from build123d import *

# Parameters (mm, degrees)
F0_W     = 50
F0_H     = 36
F1_DEPTH = 2
F2_W     = 50
F2_H     = 36
F2_W_2   = 46
F2_H_2   = 32
F3_DEPTH = 4
F4_W     = 2
F4_H     = 36
F5_DEPTH = 85
F6_W     = 50
F6_H     = 36
F7_DEPTH = 3
F8_W     = 46
F8_H     = 32
F9_DEPTH = 25


with BuildPart() as f1:
    # F0 (on Top) → F1 (new body)
    with BuildSketch(Plane.XY):
        with Locations((-32.9025480896, 24.3834912755)):
            Rectangle(F0_W, F0_H)
    extrude(amount=F1_DEPTH)

    # F2 (on face) → F3 (join)
    with BuildSketch(Plane.XY.offset(2)):
        with Locations((-32.9025480896, 24.3834912755)):
            Rectangle(F2_W, F2_H)
        with Locations((-32.9025480896, 24.3834912755)):
            Rectangle(F2_W_2, F2_H_2, mode=Mode.SUBTRACT)
    extrude(amount=F3_DEPTH)

    # F4 (on face) → F5 (join)
    with BuildSketch(Plane.XY.offset(6)):
        with Locations((-56.9025480896, 24.3834912755)):
            Rectangle(F4_W, F4_H)
        with Locations((-8.9025480896, 24.3834912755)):
            Rectangle(F4_W, F4_H)
    extrude(amount=F5_DEPTH)

    # F6 (on face) → F7 (join)
    with BuildSketch(Plane.XY.offset(91)):
        with Locations((-32.9025480896, 24.3834912755)):
            Rectangle(F6_W, F6_H)
    extrude(amount=-F7_DEPTH)

    # F8 (on face) → F9 (cut)
    with BuildSketch(Plane(origin=(0, 0, 88), x_dir=(1, 0, 0), z_dir=(0, 0, -1))):
        with Locations((-32.9025480896, -24.3834912755)):
            Rectangle(F8_W, F8_H)
    extrude(amount=-F9_DEPTH, mode=Mode.SUBTRACT)


solid = f1.part
Work out the finished part from the listing and answer in its coordinate system (mm). A direction names the side the tool comes from. Round coordinates to 2 decimals unless told otherwise and drop trailing zeros. Loops run counter-clockwise (first coordinate to the right, second up) from the corner with the lowest first, then second, coordinate; pieces in that order, holes last. Notation, with made-up numbers: (-20.5, 78.25) - (36.5, 78.25) arc R12 ccw to (36.5, 86.25) - close; hole circle Ø7 at (60, 28). An arc over 180 degrees is marked (long way). Use one line per item in the form item = value. Start each with the question number.
(1) Which of the six approach directions +Z, -Z, +X, -X, +Y, -Y give full straight-line access (tool end or side, diameter ignored) to faces 1 (the face through (-33, 7, 6)), 2 (the face through (-57, 42.383, 39)), 3 (the face through (-33, 40.383, 4))?
(2) Determine the mould class of faces 4 (the face through (-33, 40.383, 89)), 5 (the face through (-33, 25, 0)), 6 (the face through (-33, 41, 88)), 7 (the face through (-33, 41, 6)) for opening direction Z: +Z half, -Z half, draft (parallel to the pull), parting line (faces both ways), or undercut.
(3) Find section A-A on z = 80. Determine the outline of the cut face in (x, y), and give its area (3 significant figures).
(4) Flat-ended cylindrical pins translate along their axes: P1, Ø6, axis at x = -32.5, y = 30.5, coming from the -Z side; P2, Ø4, axis at x = -16.5, y = 14.5, coming from the +Z side. Find the tip coordinate at first contact, or state that the pin passes through.
(5) Find section C-C on y = 19.5. Determine the outline of the cut face in (x, z).
(6) Find section B-B on x = -29.5. Determine the outline of the cut face in (y, z), and give its area (3 significant figures).
(7) Consider line 1 (X direction, y = 21, z = 77.5); line 2 (Z direction, x = -37, y = 22). Determine where each line is inside the solid, lowest interval first.
Answer list:
q1.face_1 = +Y, -Y
q1.face_2 = +Z, -Z, +X, -X, +Y
q1.face_3 = +Z
q2.face_4 = draft
q2.face_5 = -Z half
q2.face_6 = undercut
q2.face_7 = undercut
q3.outline = (-57.9, 6.38) - (-55.9, 6.38) - (-55.9, 42.38) - (-57.9, 42.38) - close; (-9.9, 6.38) - (-7.9, 6.38) - (-7.9, 42.38) - (-9.9, 42.38) - close
q3.area = 144 mm^2
q4.P1 = 0
q4.P2 = 2
q5.outline = (-57.9, 0) - (-7.9, 0) - (-7.9, 91) - (-9.9, 91) - (-9.9, 2) - (-55.9, 2) - (-55.9, 91) - (-57.9, 91) - close
q6.outline = (6.38, 0) - (42.38, 0) - (42.38, 6) - (40.38, 6) - (40.38, 2) - (8.38, 2) - (8.38, 6) - (6.38, 6) - close; (6.38, 88) - (8.38, 88) - (8.38, 91) - (6.38, 91) - close; (40.38, 88) - (42.38, 88) - (42.38, 91) - (40.38, 91) - close
q6.area = 100 mm^2
q7.line_1 = -57.9 to -55.9, -9.9 to -7.9
q7.line_2 = 0 to 2
